Part print with two shaded views. Sizes in mm from the minimum x, y, z corner. A direction names the side the tool comes from. Coordinates: 2 decimals unless noted, no trailing zeros. Loops run counter-clockwise (first coordinate to the right, second up) from the corner with the lowest first, then second, coordinate; pieces in that order, holes last.
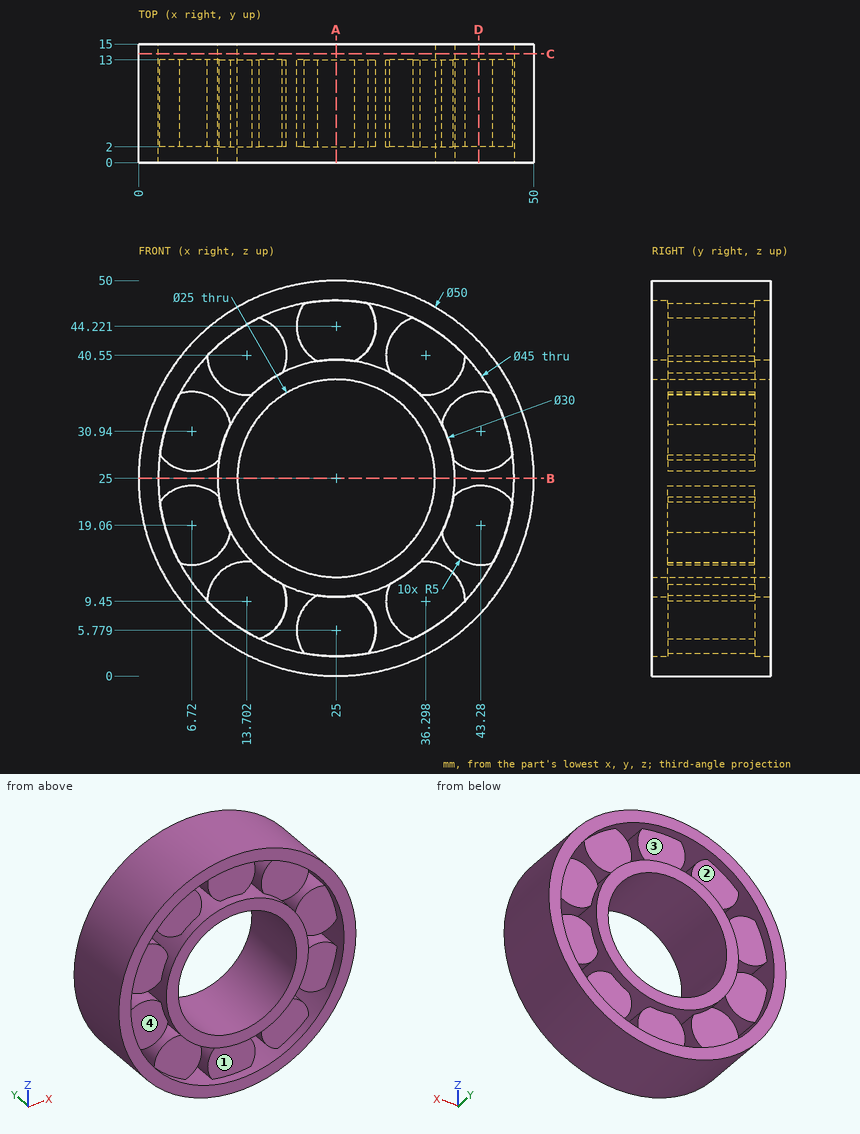
Q1. Which spindle directions (+Z, -Z, +X, -X, +Y, -Y) get a long thin tool onto all of the face, cutting with end or side? Do the marked faces 3 and 4. Say none if no direction does.
Answers:
face 3: +Y
face 4: -Y
Q2. Slice it at C-C (y = 13.75). List the corners of the cut face in (x, z), and give its area (3 significant figures).
Answers:
outline: circle Ø50 at (25, 25); circle Ø30 at (25, 25); hole circle Ø45 at (25, 25); hole circle Ø25 at (25, 25)
area: 589 mm2
Q3. Slice it at B-B (z = 25). List the corners of the cut face in (x, y).
Answers:
outline: (0, 0) - (2.5, 0) - (2.5, 15) - (0, 15) - close; (10, 0) - (12.5, 0) - (12.5, 15) - (10, 15) - close; (37.5, 0) - (40, 0) - (40, 15) - (37.5, 15) - close; (47.5, 0) - (50, 0) - (50, 15) - (47.5, 15) - close
Q4. Slice it at D-D (x = 43). List the corners of the cut face in (y, z), and give its area (3 significant figures).
Answers:
outline: (0, 7.65) - (15, 7.65) - (15, 11.5) - (0, 11.5) - close; (0, 38.5) - (15, 38.5) - (15, 42.35) - (0, 42.35) - close; (2, 14.07) - (13, 14.07) - (13, 24.05) - (2, 24.05) - close; (2, 25.95) - (13, 25.95) - (13, 35.93) - (2, 35.93) - close
area: 335 mm2
Q5. Mould opens along Y. For the marked faces 1 and 2 say: +Y half, -Y half, draft (parallel to the pull), parting line (faces both ways), or undercut.
Answers:
face 1: -Y half
face 2: +Y half
Q6. Slice it at A-A (x = 25). List the corners of the cut face in (y, z).
Answers:
outline: (0, 0) - (15, 0) - (15, 2.5) - (13, 2.5) - (13, 10) - (15, 10) - (15, 12.5) - (0, 12.5) - (0, 10) - (2, 10) - (2, 2.5) - (0, 2.5) - close; (0, 37.5) - (15, 37.5) - (15, 40) - (13, 40) - (13, 47.5) - (15, 47.5) - (15, 50) - (0, 50) - (0, 47.5) - (2, 47.5) - (2, 40) - (0, 40) - close
Q7. Flat gauge pins, fed straight in: P1, Ø3, axis at x = 34, z = 27.5, coming from the +Y side; P2, Ø2.5, axis at x = 7.5, z = 20.5, coming from the -Y side; P3, Ø4, axis at y = 6, z = 39.5, coming from the -X side; P4, Ø8, axis at y = 10.5, z = 17, coming from the -X side. Where does each tip first touch, or does it go through?
Answers:
P1: passes through
P2: stops at y = 2
P3: stops at x = 3.35
P4: stops at x = 0.32
Q8. Drill centre lines: line 1 (Z direction, x = 25, y = 4); line 2 (X direction, y = 11, z = 38) (1 decimal); line 3 (X direction, y = 11, z = 45) (1 decimal). Where is each one in solid material? Low to high.
Answers:
line 1: z = 0 to 12.5, 37.5 to 50
line 2: x = 3.6 to 6.6, 9.4 to 40.6, 43.4 to 46.4
line 3: x = 10 to 16, 20.1 to 29.9, 34 to 40
